from build123d import *

# Parameters (mm, degrees)
F0_W      = 50
F0_H      = 50
F1_DEPTH  = 25
F2_R      = 63.827171
F3_DEPTH  = 15
F1_FACE_W = 50
F1_FACE_H = 25
F4_R      = 54.988955
F4_W      = 50
F4_H      = 25
F5_DEPTH  = 15


with BuildPart() as f1:
    # F0 (on Front) → F1 (new body)
    with BuildSketch(Plane.XZ):
        Rectangle(F0_W, F0_H)
    extrude(amount=F1_DEPTH)

    # F2 (on face) → F3 (join)
    with BuildSketch(Plane.XY.offset(25)):
        with Locations((0, -10.513827)):
            Circle(F2_R)
    extrude(amount=F3_DEPTH)

    # F1_face (on face) + F4 (on face) → F5 (join)
    with BuildSketch(Plane(origin=(0, -12.5, 25), x_dir=(1, 0, 0), z_dir=(0, 0, 1))):
        Rectangle(F1_FACE_W, F1_FACE_H)
    with BuildSketch(Plane(origin=(0, 0, -25), x_dir=(1, 0, 0), z_dir=(0, 0, -1))):
        with Locations((0, 12.09332)):
            Circle(F4_R)
        with Locations((0, 12.5)):
            Rectangle(F4_W, F4_H, mode=Mode.SUBTRACT)
        with Locations((0, 12.5)):
            Rectangle(F4_W, F4_H)
    extrude(amount=F5_DEPTH)


solid = f1.part
Input: part model. Units: mm. Frame: model coordinates. A direction names the side the tool comes from. Coordinates: 2 decimals unless noted, no trailing zeros. Write each loop counter-clockwise with the first axis right and the second up, starting at its lowest first coordinate (ties: lowest second). Pieces come first, ordered by that corner, then holes. Notation, with made-up numbers: M 1,54.5 L 21,54.5 A19 ccw 21,65.5 Z; hole C 66.5,73 d9. An arc over 180 degrees is marked long. Answer as a JSON object with one key per item and string values. Group by question number.
(1) Section C-C on x = 0. Output: boundary loops of the cut face in (y, z).
(2) Section B-B on y = 16.5. Output: boundary loops of the cut face in (x, z).
(3) Section A-A on x = -46. Output: boundary loops of the cut face in (y, z).
(4) Ray query, line 1 along Z through (x, y) = (44, -19); line 2 along Y through (x, z) = (-1, -34); line 3 along X through (y, z) = (-20.5, -13.5). Return the intervals inside material, ascending. Write a range as [from, to].
(5) Mould query, pull axis Z, two halves, no side actions, for faces 6 (the face through (-1, -13, -40)), 7 (the face through (-11.92, 41.59, -32.39)), 8 (the face through (-1, -10, 40)), 9 (the face through (-1, 12, -25)). Classes: pulls with the +Z half, pulls with the -Z half, needs draft (parallel to the pull), parting line crosses it, or undercut.
(6) Section D-D on z = -17.5. Output: boundary loops of the cut face in (x, y).
(7) Set-up query: faces 1 (the face through (25, -12, 0)), 2 (the face through (-25, -12, 0)), 3 (the face through (-50.65, -49.35, 32.39)), 4 (the face through (0, -25, 0)), 5 (the face through (0, 0, 0)). Return all of +Z, -Z, +X, -X, +Y, -Y with unobstructed straight access to the full face (end or side cutting, diameter ignored); none if empty.
(8) Contact query for flat-ended pins moving along their axis: P1, Ø7.5, axis at y = -14, z = -12.5, coming from the -X side; P2, Ø25, axis at x = 6.5, z = 4, coming from the +Y side; P3, Ø12.5, axis at y = -14.5, z = -5, coming from the +X side. Output: stop coordinate, or through.
Result set:
{
 "1": {"outline": "M -74.34,25 L -25,25 L -25,-25 L -67.08,-25 L -67.08,-40 L 42.9,-40 L 42.9,-25 L 0,-25 L 0,25 L 53.31,25 L 53.31,40 L -74.34,40 Z"},
 "2": {"outline": "M -57.83,25 L 57.83,25 L 57.83,40 L -57.83,40 Z; M -46.97,-40 L 46.97,-40 L 46.97,-25 L -46.97,-25 Z"},
 "3": {"outline": "M -54.76,25 L 33.73,25 L 33.73,40 L -54.76,40 Z; M -42.22,-40 L 18.04,-40 L 18.04,-25 L -42.22,-25 Z"},
 "4": {"line 1": "z = [-40, -25], [25, 40]", "line 2": "y = [-67.07, 42.89]", "line 3": "x = [-25, 25]"},
 "5": {"face 6": "pulls with the -Z half", "face 7": "needs draft", "face 8": "pulls with the +Z half", "face 9": "undercut"},
 "6": {"outline": "M -25,-25 L 25,-25 L 25,0 L -25,0 Z"},
 "7": {"face 1": "+X, +Y, -Y", "face 2": "-X, +Y, -Y", "face 3": "+Z, -Z", "face 4": "+X, -X, -Y", "face 5": "+X, -X, +Y"},
 "8": {"P1": "stops at x = -25", "P2": "stops at y = 0", "P3": "stops at x = 25"}
}
